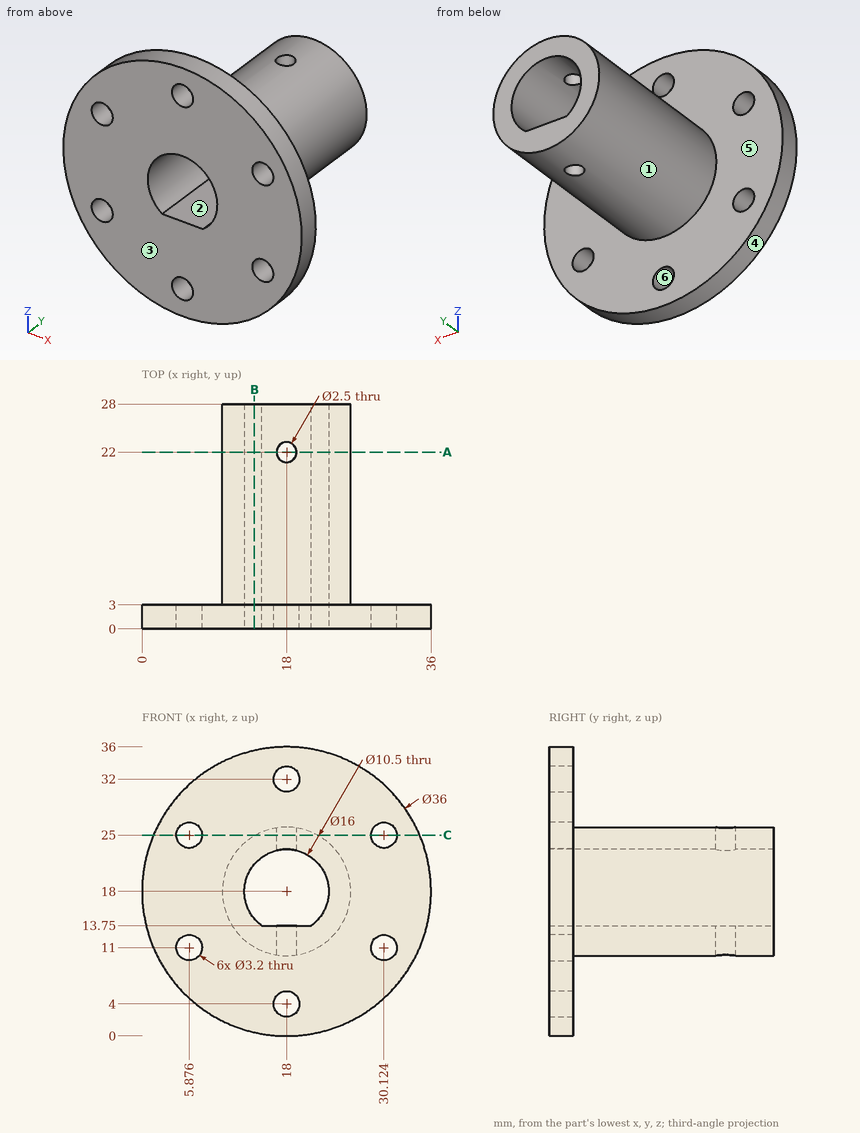
Drawing for the job (mm, zero at the part's lowest x, y, z). A direction names the side the tool comes from. Coordinates: 2 decimals unless noted, no trailing zeros. Write each loop counter-clockwise with the first axis right and the second up, starting at its lowest first coordinate (ties: lowest second). Pieces come first, ordered by that corner, then holes. Notation, with made-up numbers: (-24.5, 44) -> (8.5, 44) arc R10 cw to (8.5, 56) -> close; hole circle Ø10 at (-25.5, -14.5). An arc over 180 degrees is marked (long way). One line per item, written item: value. Start each with the question number.
1) Probe probe 1 along Y at (x, z) = (18, 10.8); probe 2 along Z at (x, y) = (18, 16.75); probe 3 along X at (y, z) = (2.25, 25) (1 decimal). List the from-to ranges inside material, lowest first.
2) Slice it at B-B on x = 14. Write the cut outline in (y, z), then the cut area to 3 significant figures.
3) Slice it at A-A on y = 22. Write the cut outline in (x, z).
4) Pull direction Z, two halves, no side cores. Call the marked faces 4, 5 and 6: +Z half, -Z half, draft (parallel to the pull), parting line (faces both ways), or undercut.
5) Flat gauge pins, fed straight in: pin 1 Ø12 at (x, y) = (15, 25) entering from -Z; pin 2 Ø4 at (x, z) = (18, 4) entering from -Y; pin 3 Ø3 at (x, y) = (18, 22) entering from +Z; pin 4 Ø12 at (x, y) = (5.5, 25) entering from -Z (1 decimal). Where does each tip first touch, or does it go through?
6) Which spindle directions (+Z, -Z, +X, -X, +Y, -Y) get a long thin tool onto all of the face, cutting with end or side? Do the marked faces 1, 2 and 3. Say none if no direction does.
7) Slice it at C-C on z = 25. Count the separate pieces of the cut face and the enclosed holes in it, then the cut area to 3 significant figures.
Answers follow:
1. probe 1: 0 to 20.75, 23.25 to 28
1. probe 2: 10 to 13.75, 23.25 to 26
1. probe 3: 1.4 to 4.3, 7.5 to 28.5, 31.7 to 34.6
2. outline: (0, 0.45) -> (3, 0.45) -> (3, 11.07) -> (28, 11.07) -> (28, 14.6) -> (0, 14.6) -> close; (0, 21.4) -> (28, 21.4) -> (28, 24.93) -> (3, 24.93) -> (3, 35.55) -> (0, 35.55) -> close
2. area: 261 mm2
3. outline: (14.92, 13.75) arc R5.25 cw to (16.75, 23.1) -> (16.75, 25.9) arc R8 ccw to (16.75, 10.1) -> (16.75, 13.75) -> close; (19.25, 10.1) arc R8 ccw to (19.25, 25.9) -> (19.25, 23.1) arc R5.25 cw to (21.08, 13.75) -> (19.25, 13.75) -> close
4. face 4: parting line
4. face 5: draft
4. face 6: undercut
5. pin 1: z = 10
5. pin 2: y = 0
5. pin 3: z = 26
5. pin 4: z = 13.3
6. face 1: +Y
6. face 2: +Y, -Y
6. face 3: +Z, -Z, +X, -X, -Y
7. separate pieces: 3
7. enclosed holes: 1
7. area: 269 mm2
